Design review of the part built by this model. Coordinates are the model's own, in mm. A direction names the side the tool comes from. Coordinates: 2 decimals unless noted, no trailing zeros. Order: outer loops, then holes, each group sorted by start corner. A loop starts at its lowest first (then second) coordinate and runs counter-clockwise, first axis right, second up. Notation, with made-up numbers: M 39.5,4.5 L 76.5,4.5 A19 cw 76.5,21.5 Z; hole C 15.25,81 d10. An arc over 180 degrees is marked long. Answer in a Markdown table with one row per item.
from build123d import *

# Parameters (mm, degrees)
SKETCH1_W           = 35.000000104
SKETCH1_H           = 25
BOSS_EXTRUDE1_DEPTH = 2
FILLET1_R           = 2.54
SKETCH2_W           = 17.220000104
SKETCH2_H           = 14.84
BOSS_EXTRUDE2_DEPTH = 4.5
FILLET2_R           = 1.27
SKETCH3_R           = 0.5
CUT_EXTRUDE1_DEPTH  = 4.5


with BuildPart() as part:
    # Sketch1 → Boss-Extrude1 (new body)
    with BuildSketch(Plane(origin=(0, 0, 0), x_dir=(1, 0, 0), z_dir=(0, 1, 0))):
        with Locations((17.500000052, 12.5)):
            Rectangle(SKETCH1_W, SKETCH1_H)
    extrude(amount=BOSS_EXTRUDE1_DEPTH)

    # Fillet1
    fillet1_edges = [part.edges().sort_by_distance(p)[0] for p in [
        (0, 1, -25),
        (35.000000104, 1, -25),
        (35.000000104, 1, 0),
        (0, 1, 0),
    ]]
    fillet(fillet1_edges, radius=FILLET1_R)

    # Sketch2 → Boss-Extrude2 (add)
    with BuildSketch(Plane(origin=(0, 2, 0), x_dir=(1, 0, 0), z_dir=(0, 1, 0))):
        with Locations((17.500000052, 12.5)):
            Rectangle(SKETCH2_W, SKETCH2_H)
    extrude(amount=BOSS_EXTRUDE2_DEPTH)

    # Fillet2
    fillet2_edges = [part.edges().sort_by_distance(p)[0] for p in [
        (8.89, 4.25, -19.92),
        (8.89, 4.25, -5.08),
        (26.110000104, 4.25, -5.08),
        (26.110000104, 4.25, -19.92),
        (8.89, 6.5, -12.5),
        (17.500000052, 6.5, -5.08),
        (26.110000104, 6.5, -12.5),
        (17.500000052, 6.5, -19.92),
    ]]
    fillet(fillet2_edges, radius=FILLET2_R)

    # Sketch3 → Cut-Extrude1 (cut)
    with BuildSketch(Plane(origin=(0, 2, 0), x_dir=(1, 0, 0), z_dir=(0, 1, 0))):
        with Locations(Location((2.54, 23.984, 0), (0, 0, 270))):
            Circle(SKETCH3_R)
        with Locations(Location((2.54, 21.444, 0), (0, 0, 270))):
            Circle(SKETCH3_R)
        with Locations(Location((2.54, 18.904, 0), (0, 0, 270))):
            Circle(SKETCH3_R)
        with Locations(Location((2.54, 16.364, 0), (0, 0, 270))):
            Circle(SKETCH3_R)
        with Locations(Location((2.54, 13.824, 0), (0, 0, 270))):
            Circle(SKETCH3_R)
        with Locations(Location((2.54, 11.284, 0), (0, 0, 270))):
            Circle(SKETCH3_R)
        with Locations(Location((2.54, 8.744, 0), (0, 0, 270))):
            Circle(SKETCH3_R)
        with Locations(Location((2.54, 6.204, 0), (0, 0, 270))):
            Circle(SKETCH3_R)
        with Locations(Location((2.54, 3.664, 0), (0, 0, 270))):
            Circle(SKETCH3_R)
        with Locations(Location((2.54, 1.124, 0), (0, 0, 270))):
            Circle(SKETCH3_R)
    extrude(amount=-CUT_EXTRUDE1_DEPTH, mode=Mode.SUBTRACT)


solid = part.part
(1) For faces 1 (the cylindrical face through (25.748, 3.638, -19.538)), 2 (the cylindrical face through (2.236, 1.014, -24.381)), 3 (the flat face through (26.11, 4, -12)), 4 (the flat face through (17, 4, -5.08)), 5 (the flat face through (17, 0, -13)), list the 3-axis set-ups (+Z, -Z, +X, -X, +Y, -Y) from which the entire face can be reached by the end or side of a thin tool; tool diameter is ignored.
Return value:
| item | result |
|---|---|
| face 1 | -Z, +X, +Y |
| face 2 | +Y, -Y |
| face 3 | +Z, -Z, +X, +Y |
| face 4 | +Z, +X, -X, +Y |
| face 5 | +Z, -Z, +X, -X, -Y |
(2) Add section A-A, the plane z = -18. Give the boundary of the cut face in (x, y).
Return value:
| item | result |
|---|---|
| outline | M 0,0 L 35,0 L 35,2 L 26.11,2 L 26.11,5.23 A1.27 ccw 24.84,6.5 L 10.16,6.5 A1.27 ccw 8.89,5.23 L 8.89,2 L 0,2 Z |
(3) For line 1 along Y through (x, z) = (4.5, -9.25); line 2 along X through (y, z) = (2.25, -17.5); line 3 along Z through (x, y) = (23, 3.75), list the stretches that pass through material, from the lowest coordinate up. Write a range as from..to.
Return value:
| item | result |
|---|---|
| line 1 | y = 0..2 |
| line 2 | x = 8.89..26.11 |
| line 3 | z = -19.92..-5.08 |
(4) Add section B-B, the plane y = 0.5. Give the number of separate pieces and of enclosed holes in the cut face, and give its area (3 significant figures).
Return value:
| item | result |
|---|---|
| separate pieces | 1 |
| enclosed holes | 10 |
| area | 862 mm2 |
(5) Add section D-D, the plane z = -21.5. Give the boundary of the cut face in (x, y), and give its area (3 significant figures).
Return value:
| item | result |
|---|---|
| outline | M 0,0 L 2.04,0 L 2.04,2 L 0,2 Z; M 3.04,0 L 35,0 L 35,2 L 3.04,2 Z |
| area | 68.0 mm2 |
(6) Draft analysis for pull direction X (two halves, no side actions). For faces 6 (the flat face through (17, 1, -25)), 7 (the cylindrical face through (2.35, 1.01, -20.98)), 8 (the cylindrical face through (9.252, 6.118, -12.586)), 9 (the cylindrical face through (25.748, 6.118, -12.586)), state which applies: pulls with the +X half, pulls with the -X half, needs draft (parallel to the pull), parting line crosses it, or undercut.
Return value:
| item | result |
|---|---|
| face 6 | needs draft |
| face 7 | undercut |
| face 8 | pulls with the -X half |
| face 9 | pulls with the +X half |
(7) Add section C-C, the plane y = 3. Give the boundary of the cut face in (x, z), and give its area (3 significant figures).
Return value:
| item | result |
|---|---|
| outline | M 8.89,-18.65 A1.27 ccw 10.16,-19.92 L 24.84,-19.92 A1.27 ccw 26.11,-18.65 L 26.11,-6.35 A1.27 ccw 24.84,-5.08 L 10.16,-5.08 A1.27 ccw 8.89,-6.35 Z |
| area | 254 mm2 |
(8) Insertion check: pin 1 Ø1 at (x, y) = (16, 4.5) entering from -Z; pin 2 Ø1.5 at (y, z) = (4.5, -14) entering from -X; pin 3 Ø4 at (x, z) = (31.5, -15) entering from +Y. Each pin has a flat end and moves straight along its axis. Give the tip position at first contact, or say it passes through.
Return value:
| item | result |
|---|---|
| pin 1 | stops at z = -19.92 |
| pin 2 | stops at x = 8.89 |
| pin 3 | stops at y = 2 |
